Could you check a few things on this model? Use its own coordinates, in mm. Face numbers are marked on the shaded views. Give positions to 0.01 mm unless a question says otherwise; leave off trailing zeros. Loops run counter-clockwise (first coordinate to the right, second up) from the corner with the lowest first, then second, coordinate; pieces in that order, holes last. Notation, with made-up numbers: (24, 64) -> (49, 64) arc R20 cw to (49, 72) -> close; hole circle Ø5 at (36.5, 47). An arc over 180 degrees is marked (long way). Write each question's results on one line, items separated by ' | '. Start each with the question number.
Q1. If we section it at B-B, the plane x = 2.5: List the corners of the cut face in (y, z) for me.
Q2. Will these pins go through, and if not, where does the flat tip stop? P1, Ø3, axis at y = 15.5, z = -7.5, coming from the -X side; P2, Ø1.5, axis at y = 11.5, z = -3.5, coming from the -X side; P3, Ø1.5, axis at x = -7.5, z = -3, coming from the +Y side.
Q3. If I drill on line 1 along Y through (x, z) = (-8, 2); line 2 along X through (y, z) = (10, 2.5); line 3 along X through (y, z) = (-1.75, 7.5), over which ranges is the centre line in solid material (lowest first)?
Q4. If we section it at C-C, the plane z = -4.5: Give the number of separate pieces and of enclosed holes in the cut face, plus the area to 3 significant figures.
Q5. We'd pull the mould along X, two halves only. Please class the marked faces 1, 2 and 3: released by +X, released by -X, zero draft, split by the parting line, or undercut.
Q6. If we section it at A-A, the plane x = -30: List the corners of the cut face in (y, z) for me, plus the area to 3 significant figures.
Q7. If we section it at D-D, the plane x = -10: List the corners of the cut face in (y, z) for me, plus the area to 3 significant figures.
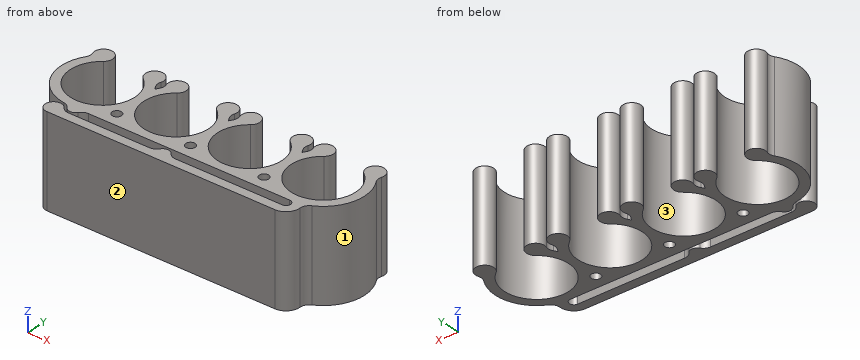
from build123d import *

# Parameters (mm, degrees)
F1_R     = 1.03125
F2_DEPTH = 10
F3_R     = 2


with BuildPart() as f2:
    # F1 (on Top) → F2 (new body, symmetric)
    with BuildSketch(Plane.XY):
        with BuildLine():
            ThreePointArc((-19.9828767123, 14.7352475904), (-17.9695529655, 12.2452360949), (-17.25, 9.125))
            ThreePointArc((-17.25, 9.125), (-27.4952360949, 2.7195529655), (-28.7671232877, 14.7352475904))
            ThreePointArc((-28.7671232877, 14.7352475904), (-29.8675330526, 18.3056622368), (-31.4302114786, 14.9120213402))
            ThreePointArc((-31.4302114786, 14.9120213402), (-32.6233996851, 5.2224972601), (-24.375, 0))
            Line((-24.375, 0), (-21.375, 0))
            Line((-21.375, 0), (24.375, 0))
            ThreePointArc((24.375, 0), (25.7175606637, 0.099305796), (27.0308996167, 0.3950617284))
            ThreePointArc((27.0308996167, 0.3950617284), (33.107808756, 6.4785540378), (31.4302114786, 14.9120213402))
            ThreePointArc((31.4302114786, 14.9120213402), (29.8675330526, 18.3056622368), (28.7671232877, 14.7352475904))
            ThreePointArc((28.7671232877, 14.7352475904), (30.7804470345, 12.2452360949), (31.5, 9.125))
            ThreePointArc((31.5, 9.125), (21.2547639051, 2.7195529655), (19.9828767123, 14.7352475904))
            ThreePointArc((19.9828767123, 14.7352475904), (18.8824669474, 18.3056622368), (17.3197885214, 14.9120213402))
            ThreePointArc((17.3197885214, 14.9120213402), (16.7410654482, 14.1238666974), (16.25, 13.2783119315))
            ThreePointArc((16.25, 13.2783119315), (15.7589345518, 14.1238666974), (15.1802114786, 14.9120213402))
            ThreePointArc((15.1802114786, 14.9120213402), (13.6175330526, 18.3056622368), (12.5171232877, 14.7352475904))
            ThreePointArc((12.5171232877, 14.7352475904), (14.5304470345, 12.2452360949), (15.25, 9.125))
            ThreePointArc((15.25, 9.125), (5.0047639051, 2.7195529655), (3.7328767123, 14.7352475904))
            ThreePointArc((3.7328767123, 14.7352475904), (2.6324669474, 18.3056622368), (1.0697885214, 14.9120213402))
            ThreePointArc((1.0697885214, 14.9120213402), (0.4910654482, 14.1238666974), (0, 13.2783119315))
            ThreePointArc((0, 13.2783119315), (-0.4910654482, 14.1238666974), (-1.0697885214, 14.9120213402))
            ThreePointArc((-1.0697885214, 14.9120213402), (-2.6324669474, 18.3056622368), (-3.7328767123, 14.7352475904))
            ThreePointArc((-3.7328767123, 14.7352475904), (-1.7195529655, 12.2452360949), (-1, 9.125))
            ThreePointArc((-1, 9.125), (-11.2452360949, 2.7195529655), (-12.5171232877, 14.7352475904))
            ThreePointArc((-12.5171232877, 14.7352475904), (-13.6175330526, 18.3056622368), (-15.1802114786, 14.9120213402))
            ThreePointArc((-15.1802114786, 14.9120213402), (-15.7589345518, 14.1238666974), (-16.25, 13.2783119315))
            ThreePointArc((-16.25, 13.2783119315), (-16.7410654482, 14.1238666974), (-17.3197885214, 14.9120213402))
            ThreePointArc((-17.3197885214, 14.9120213402), (-18.8824669474, 18.3056622368), (-19.9828767123, 14.7352475904))
        make_face()
        with Locations((-16.25, 3.03125)):
            Circle(F1_R, mode=Mode.SUBTRACT)
        with Locations((0, 3.03125)):
            Circle(F1_R, mode=Mode.SUBTRACT)
        with Locations((16.25, 3.03125)):
            Circle(F1_R, mode=Mode.SUBTRACT)
        with BuildLine():
            ThreePointArc((27.0308996167, 0.3950617284), (25.7175606637, 0.099305796), (24.375, 0))
            ThreePointArc((24.375, 0), (25.375, -1), (24.375, -2))
            Line((24.375, -2), (-0.6061253537, -2))
            Line((-0.6061253537, -2), (-3.6061253537, -2))
            Line((-3.6061253537, -2), (-24.1903478035, -2))
            ThreePointArc((-24.1903478035, -2), (-27.3314384085, -0.985167759), (-25.9871463178, -4))
            Line((-25.9871463178, -4), (24.375, -4))
            ThreePointArc((24.375, -4), (26.9426044463, -2.5515822271), (27.0308996167, 0.3950617284))
        make_face()
        with BuildLine():
            Line((-21.375, 0), (-24.375, 0))
            ThreePointArc((-24.375, 0), (-22.875, -1.5), (-21.375, 0))
        make_face()
        with BuildLine():
            Line((-3.6061253537, -2), (-0.6061253537, -2))
            ThreePointArc((-0.6061253537, -2), (-2.1061253537, -0.5), (-3.6061253537, -2))
        make_face()
    extrude(amount=F2_DEPTH, both=True)

    # F3
    f3_edges = [f2.edges().sort_by_distance(p)[0] for p in [
        (31.430211, 14.912021, 0),
        (15.180211, 14.912021, 0),
        (17.319789, 14.912021, 0),
        (1.069789, 14.912021, 0),
        (-15.180211, 14.912021, 0),
        (-31.430211, 14.912021, 0),
        (-17.319789, 14.912021, 0),
        (-1.069789, 14.912021, 0),
        (-24.375, 0, 0),
        (27.0309, 0.395062, 0),
        (-24.190348, -2, 0),
        (-0.606125, -2, 0),
        (-3.606125, -2, 0),
        (-21.375, 0, 0),
    ]]
    fillet(f3_edges, radius=F3_R)


solid = f2.part
Final values:
1) outline: (-4, -10) -> (-2, -10) -> (-2, 10) -> (-4, 10) -> close; (0, -10) -> (4.75, -10) -> (4.75, 10) -> (0, 10) -> close; (13.5, -10) -> (18.31, -10) -> (18.31, 10) -> (13.5, 10) -> close
2) P1: stops at x = -32.09 | P2: stops at x = -33.35 | P3: stops at y = 2.13
3) line 1: y = -4 to -2, 0 to 2 | line 2: x = -33.46 to -31.45, -17.3 to -15.2, -1.05 to 1.05, 15.2 to 17.3, 31.45 to 33.46 | line 3: x = -27.74 to -23.84, -4.01 to -0.2, 25.04 to 27.28
4) separate pieces: 1 | enclosed holes: 3 | area: 552 mm²
5) face 1: released by +X | face 2: zero draft | face 3: undercut
6) outline: (1.94, -10) -> (4.75, -10) -> (4.75, 10) -> (1.94, 10) -> close; (13.5, -10) -> (18.31, -10) -> (18.31, 10) -> (13.5, 10) -> close | area: 152 mm²
7) outline: (-4, -10) -> (-2, -10) -> (-2, 10) -> (-4, 10) -> close; (0, -10) -> (2.25, -10) -> (2.25, 10) -> (0, 10) -> close | area: 85.0 mm²
